Study the drawing (mm; zero at the part's minimum x, y, z) and answer. A direction names the side the tool comes from. Round coordinates to 2 decimals unless told otherwise and drop trailing zeros. Loops run counter-clockwise (first coordinate to the right, second up) from the corner with the lowest first, then second, coordinate; pieces in that order, holes last. Notation, with made-up numbers: M 34.5,41 L 49.5,41 A35 cw 49.5,80 Z; hole C 80,10 d10. An arc over 180 degrees is marked long. Put each result on its own line as item: value. Start each with the question number.
(1) Straight lines are drawn through the part: line 1 (Y direction, x = 7.25, z = 0.3) (1 decimal); line 2 (Z direction, x = 5.25, y = 6); line 3 (Y direction, x = 6, z = 1.75) (1 decimal). For each, find the intervals that lie inside material, in ascending order.
(2) Section C-C, the plane y = 6 is taken. Determine the outline of the cut face in (x, z) (1 decimal), then the cut area to 3 significant figures.
(3) Which of the six approach directions +Z, -Z, +X, -X, +Y, -Y give full straight-line access (tool end or side, diameter ignored) to the marked faces 1 and 2?
(4) Section A-A, the plane x = 6 is taken. Determine the outline of the cut face in (y, z) (1 decimal), then the cut area to 3 significant figures.
(5) Determine the mould class of the marked faces 3, 4 and 5 for opening direction Y: released by +Y, released by -Y, zero draft, split by the parting line, or undercut.
(6) Flat-ended cylindrical pins translate along their axes: P1, Ø4, axis at x = 4, y = 6, coming from the +Z side; P2, Ø1, axis at x = 7.5, z = 2, coming from the +Y side; P3, Ø2, axis at x = 8.5, y = 6.5, coming from the -Z side; P4, Ø1, axis at x = 4.5, z = 2, coming from the -Y side. Find the tip coordinate at first contact, or state that the pin passes through.
(7) Section B-B, the plane z = 1.65 is taken. Determine the outline of the cut face in (x, y) (1 decimal).
(8) Section D-D, the plane y = 4 is taken. Count the separate pieces of the cut face and the enclosed holes in it, then the cut area to 3 significant figures.
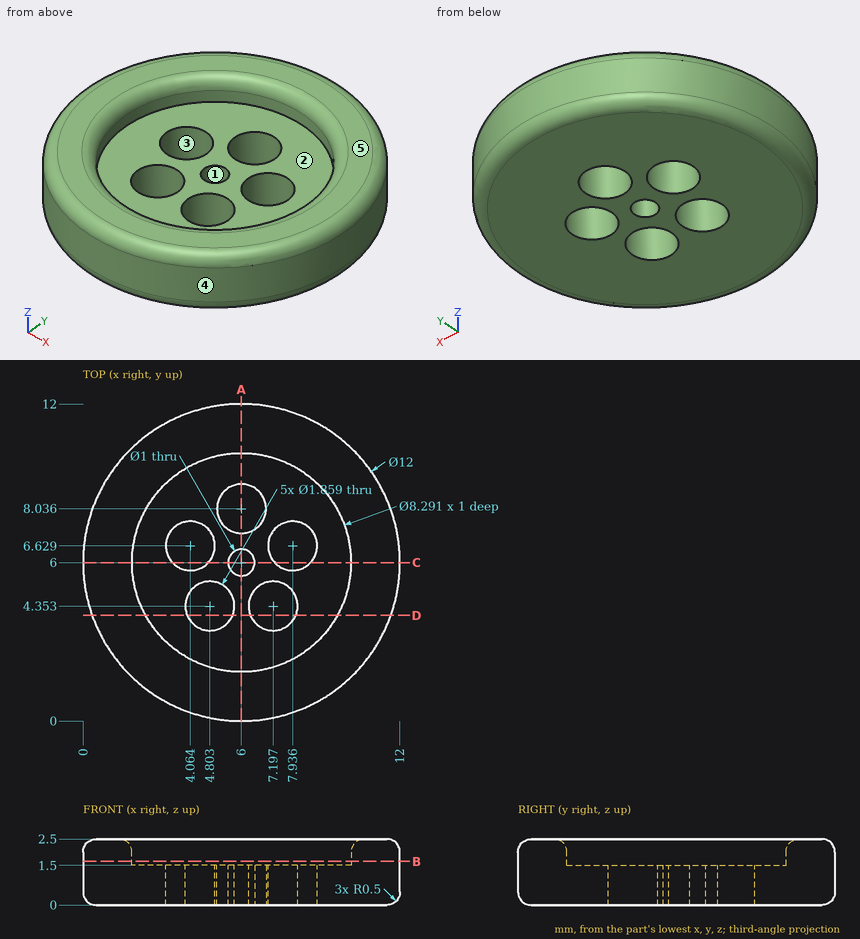
Recorded:
1. line 1: y = 0.2 to 3.4, 5.3 to 6, 7.3 to 11.8
1. line 2: z = 0 to 1.5
1. line 3: y = 0 to 1.9, 10.1 to 12
2. outline: M 0,0.5 A0.5 ccw 0.5,0 L 3.4,0 L 3.4,1.5 L 1.9,1.5 L 1.9,2 A0.5 ccw 1.4,2.5 L 0.5,2.5 A0.5 ccw 0,2 Z; M 4.7,0 L 5.5,0 L 5.5,1.5 L 4.7,1.5 Z; M 6.5,0 L 7.3,0 L 7.3,1.5 L 6.5,1.5 Z; M 8.6,0 L 11.5,0 A0.5 ccw 12,0.5 L 12,2 A0.5 ccw 11.5,2.5 L 10.6,2.5 A0.5 ccw 10.1,2 L 10.1,1.5 L 8.6,1.5 Z
2. area: 15.8 mm²
3. face 1: +Z, -Z
3. face 2: +Z
4. outline: M 0,0.5 A0.5 ccw 0.5,0 L 5.5,0 L 5.5,1.5 L 1.9,1.5 L 1.9,2 A0.5 ccw 1.4,2.5 L 0.5,2.5 A0.5 ccw 0,2 Z; M 6.5,0 L 7.1,0 L 7.1,1.5 L 6.5,1.5 Z; M 9,0 L 11.5,0 A0.5 ccw 12,0.5 L 12,2 A0.5 ccw 11.5,2.5 L 10.6,2.5 A0.5 ccw 10.1,2 L 10.1,1.5 L 9,1.5 Z
4. area: 17.1 mm²
5. face 3: undercut
5. face 4: split by the parting line
5. face 5: zero draft
6. P1: stops at z = 1.5
6. P2: stops at y = 11.92
6. P3: stops at z = 0
6. P4: stops at y = 0.08
7. outline: C 6,6 d12; hole C 6,6 d8.3
8. separate pieces: 3
8. enclosed holes: 0
8. area: 15.5 mm²
